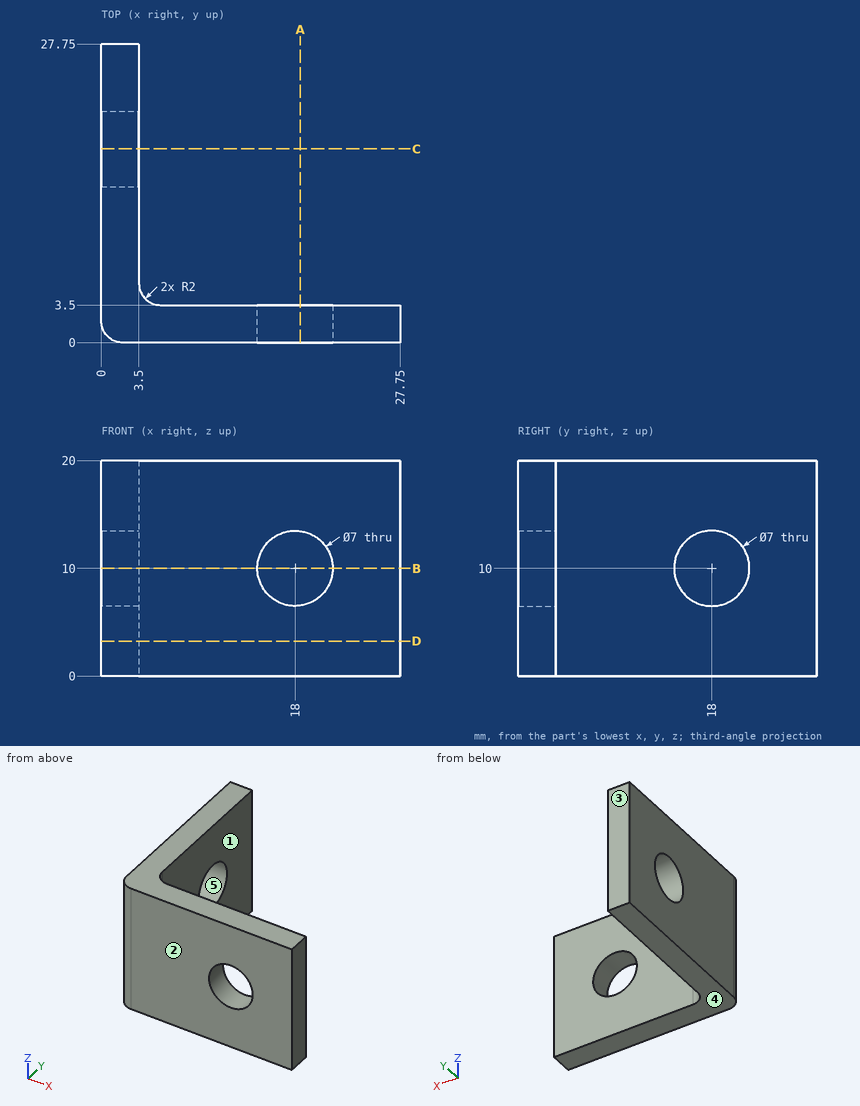
Geometry check sheet. Reference: drawing and pictorial views, mm from the part's lowest x, y, z. A direction names the side the tool comes from. Round coordinates to 2 decimals unless told otherwise and drop trailing zeros. Order: outer loops, then holes, each group sorted by start corner. A loop starts at its lowest first (then second) coordinate and runs counter-clockwise, first axis right, second up. Notation, with made-up numbers: (52.5, 59.5) - (69.5, 59.5) arc R34 ccw to (69.5, 92.5) - close; hole circle Ø3 at (33.5, -30). An arc over 180 degrees is marked (long way). One line per question, with ' | ' between items. Start each with the question number.
(1) Access from +Z, -Z, +X, -X, +Y, -Y to the whole of each face (thin tool, end or side, straight path). Record for the marked faces 1 and 2.
(2) Sectioned sample at B-B on z = 10. Record the cut outline in (x, y), and give its area (3 significant figures).
(3) Sectioned sample at C-C on y = 18. Record the cut outline in (x, z), and give its area (3 significant figures).
(4) Sectioned sample at A-A on x = 18.5. Record the cut outline in (y, z), and give its area (3 significant figures).
(5) Sectioned sample at D-D on z = 3.25. Record the cut outline in (x, y), and give its area (3 significant figures).
(6) Release check for a two-part mould opening along Y. For the marked faces 3, 4 and 5 record: released by +Y, released by -Y, zero draft, split by the parting line, or undercut.
(7) Thickness scan on L1, parallel to Y at x = 2.35, z = 10; L2, parallel to Y at x = 21.75, z = 14. Record the ranges inside material, lowest first. Write a range as [from, to].
(8) Depth check by flat-ended pin: pin 1 Ø6 at (y, z) = (16, 13.5) entering from +X; pin 2 Ø8 at (x, z) = (18, 10) entering from +Y. Enter the tip coordinate at first touch or a pass-through.
Conclusion:
1) face 1: +Z, -Z, +X, +Y | face 2: +Z, -Z, +X, -X, -Y
2) outline: (0, 2) arc R2 ccw to (2, 0) - (14.5, 0) - (14.5, 3.5) - (5.5, 3.5) arc R2 cw to (3.5, 5.5) - (3.5, 14.5) - (0, 14.5) - close; (0, 21.5) - (3.5, 21.5) - (3.5, 27.75) - (0, 27.75) - close; (21.5, 0) - (27.75, 0) - (27.75, 3.5) - (21.5, 3.5) - close | area: 133 mm2
3) outline: (0, 0) - (3.5, 0) - (3.5, 6.5) - (0, 6.5) - close; (0, 13.5) - (3.5, 13.5) - (3.5, 20) - (0, 20) - close | area: 45.5 mm2
4) outline: (0, 0) - (3.5, 0) - (3.5, 6.54) - (0, 6.54) - close; (0, 13.46) - (3.5, 13.46) - (3.5, 20) - (0, 20) - close | area: 45.8 mm2
5) outline: (0, 2) arc R2 ccw to (2, 0) - (27.75, 0) - (27.75, 3.5) - (5.5, 3.5) arc R2 cw to (3.5, 5.5) - (3.5, 27.75) - (0, 27.75) - close | area: 182 mm2
6) face 3: released by +Y | face 4: zero draft | face 5: undercut
7) L1: y = [0, 14.5], [21.5, 27.75] | L2: y = [0, 3.5]
8) pin 1: stops at x = 3.5 | pin 2: stops at y = 3.5
